Geometry: final body of the model. Coordinates: model frame, mm. Face numbers are marked on the shaded views. A direction names the side the tool comes from. Coordinates: 2 decimals unless noted, no trailing zeros. Loops run counter-clockwise (first coordinate to the right, second up) from the corner with the lowest first, then second, coordinate; pieces in that order, holes last. Notation, with made-up numbers: M -7,-3.75 L 39,-3.75 A22 cw 39,26.25 Z; hole C 12.25,38.5 d11. An arc over 180 degrees is marked long. Write item = value, one per line. Start each with the question number.
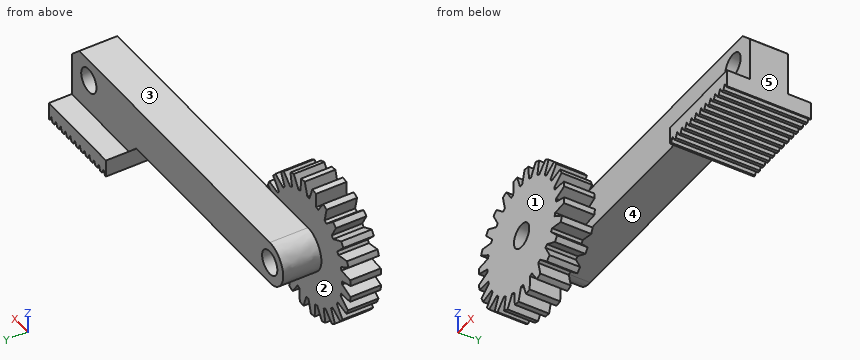
```python
from build123d import *

# Parameters (mm, degrees)
ESQUISSE1_R                  = 9
BOSS_EXTRU_1_DEPTH           = 4
BOSS_EXTRU_2_DEPTH           = 5
ENL_V_MAT_EXTRU_1_DEPTH      = 10
ENL_V_MAT_EXTRU_1_DEPTH_BACK = 12
ESQUISSE3_R                  = 1.6
ENL_V_MAT_EXTRU_2_DEPTH      = 4
BOSS_EXTRU_3_DEPTH           = 3
BOSS_EXTRU_3_DEPTH_BACK      = 8
ESQUISSE5_W                  = 12
ESQUISSE5_H                  = 2.28739505
ENL_V_MAT_EXTRU_3_DEPTH      = 11
ESQUISSE7_R                  = 1.6
ENL_V_MAT_EXTRU_4_DEPTH      = 11


with BuildPart() as part:
    # Esquisse1 → Boss.-Extru.1 (new body)
    with BuildSketch(Plane(origin=(0, 0, 0), x_dir=(1, 0, 0), z_dir=(0, 1, 0))):
        with Locations(Location((0, 0, 0), (0, 0, 270))):
            Circle(ESQUISSE1_R)
    extrude(amount=BOSS_EXTRU_1_DEPTH)

    # Esquisse2 → Boss.-Extru.2 (add)
    with BuildSketch(Plane(origin=(0, 4, 0), x_dir=(1, 0, 0), z_dir=(0, 1, 0))):
        with BuildLine():
            Line((0, 2.856302475), (28, 2.856302475))
            Line((28, 2.856302475), (29.582547561, 4.38455089))
            Line((29.582547561, 4.38455089), (29.582547561, 6.67194594))
            Line((29.582547561, 6.67194594), (41.582547561, 6.67194594))
            Line((41.582547561, 6.67194594), (41.582547561, -1.32805406))
            Line((41.582547561, -1.32805406), (40, -2.856302475))
            Line((40, -2.856302475), (28, -2.856302475))
            Line((28, -2.856302475), (0, -2.856302475))
            add(Edge.make_bspline(
                [(0, 2.856302475), (-1.606608321, 2.917963895), (-4.109305793, 0.012086108), (-1.551274166, -2.952682253), (0, -2.856302475)],
                knots=[0, 0, 0, 0, 0.499550893, 1, 1, 1, 1], degree=3))
        make_face()
    extrude(amount=BOSS_EXTRU_2_DEPTH)

    # Esquisse3 → Enlèv. mat.-Extru.1 (cut, two sides: drawn at the far end of the back side and taken through both)
    with BuildSketch(Plane(origin=(0, 9, 0), x_dir=(1, 0, 0), z_dir=(0, 1, 0)).offset(-ENL_V_MAT_EXTRU_1_DEPTH_BACK)):
        with Locations(Location((0, 0, 0), (0, 0, 90))):
            Circle(ESQUISSE3_R)
    extrude(amount=ENL_V_MAT_EXTRU_1_DEPTH + ENL_V_MAT_EXTRU_1_DEPTH_BACK, mode=Mode.SUBTRACT)

    # Esquisse4 → Enlèv. mat.-Extru.2 (cut)
    with BuildSketch(Plane.XZ):
        Polygon((-1.417985005, -8.887593517), (-1.548540755, -7.052961635), (-1.968711567, -6.928820259), (-2.948701489, -8.503244059), (-2.361037532, -9.099305947), align=None)
        Polygon((-3.669946805, -8.217754587), (-3.321216304, -6.411845955), (-3.69493999, -6.183186386), (-5.04902843, -7.45032294), (-4.635660805, -8.178173136), align=None)
        Polygon((-5.671807795, -6.987889262), (-4.86755645, -5.33377357), (-5.169364359, -5.016178579), (-6.805272427, -5.889674625), (-6.594371455, -6.699711341), align=None)
        Polygon((-7.287144457, -5.281810832), (-6.082180668, -3.892213331), (-6.291505089, -3.507326492), (-8.097748355, -3.927654717), (-8.103686589, -4.76467529), align=None)
        Polygon((-8.405874267, -3.215785722), (-6.882314325, -2.185405185), (-6.984890145, -1.7594559), (-8.838376114, -1.697971632), (-9.060748873, -2.504934491), align=None)
        Polygon((-8.951757637, -0.93061013), (-7.213429634, -0.329665287), (-7.202266481, 0.108318704), (-8.976683148, 0.647425415), (-9.400336095, -0.074486547), align=None)
        Polygon((-8.887593517, 1.417985005), (-7.052961635, 1.548540755), (-6.928820259, 1.968711567), (-8.503244059, 2.948701489), (-9.099305947, 2.361037532), align=None)
        Polygon((-8.217754587, 3.669946805), (-6.411845955, 3.321216304), (-6.183186386, 3.69493999), (-7.45032294, 5.04902843), (-8.178173136, 4.635660805), align=None)
        Polygon((-6.987889262, 5.671807795), (-5.33377357, 4.86755645), (-5.016178579, 5.169364359), (-5.889674625, 6.805272427), (-6.699711341, 6.594371455), align=None)
        Polygon((-5.281810832, 7.287144457), (-3.892213331, 6.082180668), (-3.507326492, 6.291505089), (-3.927654717, 8.097748355), (-4.76467529, 8.103686589), align=None)
        Polygon((-3.215785722, 8.405874267), (-2.185405185, 6.882314325), (-1.7594559, 6.984890145), (-1.697971632, 8.838376114), (-2.504934491, 9.060748873), align=None)
        Polygon((-0.93061013, 8.951757637), (-0.329665287, 7.213429634), (0.108318704, 7.202266481), (0.647425415, 8.976683148), (-0.074486547, 9.400336095), align=None)
        Polygon((1.417985005, 8.887593517), (1.548540755, 7.052961635), (1.968711567, 6.928820259), (2.948701489, 8.503244059), (2.361037532, 9.099305947), align=None)
        Polygon((3.669946805, 8.217754587), (3.321216304, 6.411845955), (3.69493999, 6.183186386), (5.04902843, 7.45032294), (4.635660805, 8.178173136), align=None)
        Polygon((5.671807795, 6.987889262), (4.86755645, 5.33377357), (5.169364359, 5.016178579), (6.805272427, 5.889674625), (6.594371455, 6.699711341), align=None)
        Polygon((7.287144457, 5.281810832), (6.082180668, 3.892213331), (6.291505089, 3.507326492), (8.097748355, 3.927654717), (8.103686589, 4.76467529), align=None)
        Polygon((8.405874267, 3.215785722), (6.882314325, 2.185405185), (6.984890145, 1.7594559), (8.838376114, 1.697971632), (9.060748873, 2.504934491), align=None)
        Polygon((8.951757637, 0.93061013), (7.213429634, 0.329665287), (7.202266481, -0.108318704), (8.976683148, -0.647425415), (9.400336095, 0.074486547), align=None)
        Polygon((8.887593517, -1.417985005), (7.052961635, -1.548540755), (6.928820259, -1.968711567), (8.503244059, -2.948701489), (9.099305947, -2.361037532), align=None)
        Polygon((8.217754587, -3.669946805), (6.411845955, -3.321216304), (6.183186386, -3.69493999), (7.45032294, -5.04902843), (8.178173136, -4.635660805), align=None)
        Polygon((6.987889262, -5.671807795), (5.33377357, -4.86755645), (5.016178579, -5.169364359), (5.889674625, -6.805272427), (6.699711341, -6.594371455), align=None)
        Polygon((5.281810832, -7.287144457), (3.892213331, -6.082180668), (3.507326492, -6.291505089), (3.927654717, -8.097748355), (4.76467529, -8.103686589), align=None)
        Polygon((3.215785722, -8.405874267), (2.185405185, -6.882314325), (1.7594559, -6.984890145), (1.697971632, -8.838376114), (2.504934491, -9.060748873), align=None)
        Polygon((0.93061013, -8.951757637), (0.329665287, -7.213429634), (-0.108318704, -7.202266481), (-0.647425415, -8.976683148), (0.074486547, -9.400336095), align=None)
    extrude(amount=-ENL_V_MAT_EXTRU_2_DEPTH, mode=Mode.SUBTRACT)

    # Esquisse5 → Boss.-Extru.3 (add, two sides: drawn at the far end of the back side and taken through both)
    with BuildSketch(Plane(origin=(0, 9, 0), x_dir=(1, 0, 0), z_dir=(0, 1, 0)).offset(-BOSS_EXTRU_3_DEPTH_BACK)):
        with Locations((35.582547561, 5.528248415)):
            Rectangle(ESQUISSE5_W, ESQUISSE5_H)
    extrude(amount=BOSS_EXTRU_3_DEPTH + BOSS_EXTRU_3_DEPTH_BACK)

    # Esquisse6 → Enlèv. mat.-Extru.3 (cut)
    with BuildSketch(Plane(origin=(0, 12, 0), x_dir=(1, 0, 0), z_dir=(0, 1, 0))):
        Polygon((41.432080312, 6.67194594), (41.097414224, 6.023830859), (40.799482778, 6.67194594), (41.122702548, 7.12855331), align=None)
        Polygon((40.432080312, 6.67194594), (40.097414224, 6.023830859), (39.799482778, 6.67194594), (40.122702548, 7.12855331), align=None)
        Polygon((39.432080312, 6.67194594), (39.097414224, 6.023830859), (38.799482778, 6.67194594), (39.097414224, 7.165876079), align=None)
        Polygon((38.432080312, 6.67194594), (38.097414224, 6.023830859), (37.799482778, 6.67194594), (38.205026004, 7.165876079), align=None)
        Polygon((37.432080312, 6.67194594), (37.097414224, 6.023830859), (36.799482778, 6.67194594), (37.097414224, 7.165876079), align=None)
        Polygon((36.432080312, 6.67194594), (36.097414224, 6.023830859), (35.799482778, 6.67194594), (36.097414224, 7.165876079), align=None)
        Polygon((35.432080312, 6.67194594), (35.097414224, 6.023830859), (34.799482778, 6.67194594), (35.097414224, 7.165876079), align=None)
        Polygon((34.432080312, 6.67194594), (34.097414224, 6.023830859), (33.799482778, 6.67194594), (34.205026004, 7.165876079), align=None)
        Polygon((33.432080312, 6.67194594), (33.097414224, 6.023830859), (32.799482778, 6.67194594), (33.205026004, 7.165876079), align=None)
        Polygon((32.432080312, 6.67194594), (32.097414224, 6.023830859), (31.799482778, 6.67194594), (32.209344848, 7.15648094), align=None)
        Polygon((31.432080312, 6.67194594), (31.097414224, 6.023830859), (30.799482778, 6.67194594), (31.097414224, 6.955035779), align=None)
        Polygon((30.432080312, 6.67194594), (30.097414224, 6.023830859), (29.799482778, 6.67194594), (30.166939204, 7.248729466), align=None)
    extrude(amount=-ENL_V_MAT_EXTRU_3_DEPTH, mode=Mode.SUBTRACT)

    # Esquisse7 → Enlèv. mat.-Extru.4 (cut)
    with BuildSketch(Plane(origin=(0, 9, 0), x_dir=(1, 0, 0), z_dir=(0, 1, 0))):
        with Locations(Location((38, 0, 0), (0, 0, 270))):
            Circle(ESQUISSE7_R)
    extrude(amount=-ENL_V_MAT_EXTRU_4_DEPTH, mode=Mode.SUBTRACT)


solid = part.part
```
Item 1: Line query: line 1 (X direction, y = 7.85, z = 0); line 2 (X direction, y = 3.5, z = -8); line 3 (X direction, y = 2.75, z = 7.5). Output: solid intervals per line, ascending. Write a range as from..to.
Item 2: Reachability of the marked faces 1, 2 and 3 from +Z, -Z, +X, -X, +Y, -Y: full face, straight path, thin tool, end or side. Return the list, or none.
Item 3: Section query B-B (x = 22). Return the cut outline in (y, z), plus the area to 3 significant figures.
Item 4: First-contact query: pin 1 (3.5 mm diameter, centred on x = 33, y = 3, fed in from +Z); pin 2 (10 mm diameter, centred on x = 16, z = -1.5, fed in from +Y); pin 3 (1.5 mm diameter, centred on x = 14, z = 1, fed in from -Y). Flat tips, straight axial feed; report the tip coordinate or a pass-through.
Item 5: Pull-direction query (X, two-part tool) for the marked faces 4 and 5; classes: released by +X, released by -X, zero draft, split by the parting line, or undercut.
Item 6: Section query A-A (y = 7.5). Count the separate pieces of the cut face and the enclosed holes in it, plus the area to 3 significant figures.
Verdict:
q1.line_1 = -2.84..-1.6, 1.6..36.4, 39.6..41.58
q1.line_2 = -3.63..-2.64, -1.48..-0.35, 0.6..1.73, 2.94..3.9
q1.line_3 = -3.79..-2.6, -1.74..-0.43, 0.2..1.52, 2.32..3.53
q2.face_1 = +Z, -Z, +X, -X, -Y
q2.face_2 = -X, +Y
q2.face_3 = +Z, +X, -X, +Y
q3.outline = M 4,-2.86 L 9,-2.86 L 9,2.86 L 4,2.86 Z
q3.area = 28.6 mm2
q4.pin_1 = 2.86
q4.pin_2 = 9
q4.pin_3 = 4
q5.face_4 = zero draft
q5.face_5 = released by +X
q6.separate_pieces = 1
q6.enclosed_holes = 2
q6.area = 278 mm2
